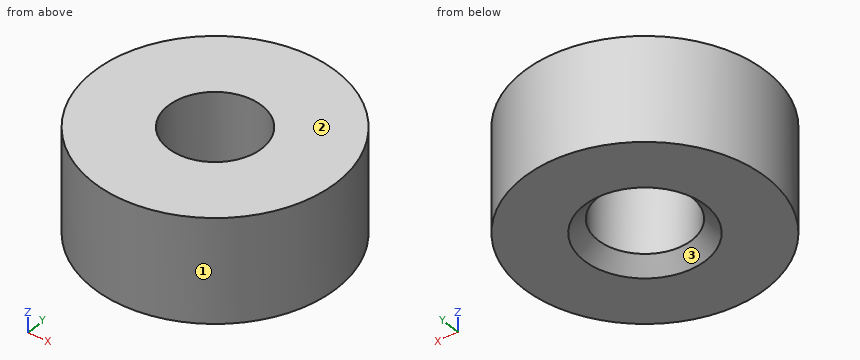
```python
from build123d import *

# Parameters (mm, degrees)
CYLINDER001_R     = 1.35
CYLINDER001_DEPTH = 3
CYLINDER_R        = 3.5
CYLINDER_DEPTH    = 3
CHAMFER_SIZE      = 0.4


with BuildPart() as cylinder001:
    # Cylinder001 → Cylinder001 (new body)
    with BuildSketch(Plane.XY):
        Circle(CYLINDER001_R)
    extrude(amount=CYLINDER001_DEPTH)


with BuildPart() as chamfer_body:
    # Cylinder → Cylinder (new body)
    with BuildSketch(Plane.XY):
        Circle(CYLINDER_R)
    extrude(amount=CYLINDER_DEPTH)

    # Cut: cut Cylinder001
    add(cylinder001.part, mode=Mode.SUBTRACT)

    # Chamfer
    chamfer_edges = [chamfer_body.edges().sort_by_distance(p)[0] for p in [
        (-1.35, 0, 0),
    ]]
    chamfer(chamfer_edges, length=CHAMFER_SIZE)


solid = chamfer_body.part
```
Design review of the part built by this model. Coordinates are the model's own, in mm. Face numbers are marked on the shaded views. Coordinates: 2 decimals unless noted, no trailing zeros. Order: outer loops, then holes, each group sorted by start corner. A loop starts at its lowest first (then second) coordinate and runs counter-clockwise, first axis right, second up. Notation, with made-up numbers: (44, 89) -> (100, 89) arc R8 ccw to (100, 97) -> close; hole circle Ø5 at (-37.75, 15.25). An arc over 180 degrees is marked (long way). One line per item, written item: value. Start each with the question number.
Q1. Insertion check: pin 1 Ø1.5 at (y, z) = (2.5, 2.5) entering from -X; pin 2 Ø3 at (x, y) = (0, 0) entering from -Z; pin 3 Ø1 at (x, z) = (0.5, 0.5) entering from -Y. Each pin has a flat end and moves straight along its axis. Give the tip position at first contact, or say it passes through.
Q2. Take a section at D-D, the plane y = 2.25. State the section outline as (x, z) points, then the cut area to 3 significant figures.
Q3. Take a section at C-C, the plane z = 2.55. State the section outline as (x, y) points, then the cut area to 3 significant figures.
Q4. Mouldability with a two-part tool opening along Y and no side actions: class the marked faces 1, 2 and 3 as pulls with the +Y half, pulls with the -Y half, needs draft (parallel to the pull), parting line crosses it, or undercut.
Q5. Take a section at A-A, the plane x = 0. State the section outline as (y, z) points, then the cut area to 3 significant figures.
Q6. For probe 1 along Y at (x, z) = (0, 2.25); probe 2 along Y at (x, z) = (-1.5, 1.95); probe 3 along Y at (x, z) = (2.75, 2.05), list the stretches that pass through material, from the lowest coordinate up.
Values follow:
1. pin 1: stops at x = -3.03
1. pin 2: stops at z = 0.25
1. pin 3: stops at y = -3.5
2. outline: (-2.68, 0) -> (2.68, 0) -> (2.68, 3) -> (-2.68, 3) -> close
2. area: 16.1 mm2
3. outline: circle Ø7 at (0, 0); hole circle Ø2.7 at (0, 0)
3. area: 32.8 mm2
4. face 1: parting line crosses it
4. face 2: needs draft
4. face 3: undercut
5. outline: (-3.5, 0) -> (-1.75, 0) -> (-1.35, 0.4) -> (-1.35, 3) -> (-3.5, 3) -> close; (1.35, 0.4) -> (1.75, 0) -> (3.5, 0) -> (3.5, 3) -> (1.35, 3) -> close
5. area: 12.7 mm2
6. probe 1: y = -3.5 to -1.35, 1.35 to 3.5
6. probe 2: y = -3.16 to 3.16
6. probe 3: y = -2.17 to 2.17
